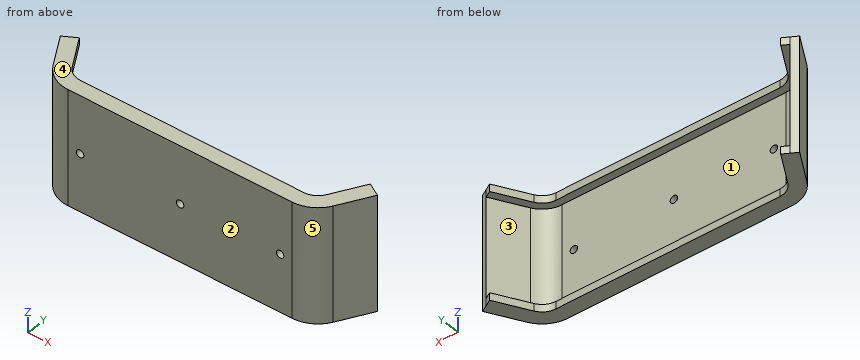
Autodesk Inventor part; units mm, degrees
ref_plane "Work Plane2" through (0, 0, 20) normal (0, 0, 1) x (1, 0, 0)
ref_plane "YZ Plane" through (0, 0, 0) normal (1, 0, 0) x (0, 1, 0)
ref_plane "XZ Plane" through (0, 0, 0) normal (0, 1, 0) x (-1, 0, 0)
sketch "Sketch1" plane through (0, 0, 0) normal (0, 0, 1) x (1, 0, 0)
  arc A0 (-53.4049, 8) -> (-44.7446, 3) centre (-44.7446, 13) ccw
  line L0 (-44.7446, 3) -> (44.7446, 3)
  arc A1 (44.7446, 3) -> (53.4049, 8) centre (44.7446, 13) ccw
  line L1 (53.4049, 8) -> (60.8108, 20.8273)
  line L2 (-60.8108, 20.8273) -> (-53.4049, 8)
  line L3 (63.4088, 19.3273) -> (56.003, 6.5)
  arc A2 (44.7446, 0) -> (56.003, 6.5) centre (44.7446, 13) ccw
  line L4 (44.7446, 0) -> (-44.7446, 0)
  arc A3 (-56.003, 6.5) -> (-44.7446, 0) centre (-44.7446, 13) ccw
  line L5 (-56.003, 6.5) -> (-63.4088, 19.3273)
  line L6 (-63.4088, 19.3273) -> (-60.8108, 20.8273)
  line L7 (-60.8108, 20.8273) -> (60.8108, 20.8273) construction
  line L8 (-63.4088, 19.3273) -> (63.4088, 19.3273) construction
  line L9 (60.8108, 20.8273) -> (63.4088, 19.3273)
  point P0 (0, 0)
  point P1 (0, 0)
extrude "Extrusion1" add sketch "Sketch1" along normal blind 40
sketch "Sketch2" plane through (-44.7446, 0, 0) normal (0, -1, 0) x (1, 0, 0)
  line L0 (89.4893, 0) -> (0, 0)
  line L1 (-11.2583, 0) -> (-11.2583, 40)
  line L2 (0, 0) -> (0, 40)
  line L3 (89.4893, 0) -> (89.4893, 40)
  point P0 (44.7446, 0)
  point P1 (4.7446, 20)
  point P2 (44.7446, 20)
  point P3 (84.7446, 20)
  point P4 (44.7446, 0)
  point P5 (-11.2583, 20)
  dimension "d3" = 40
  dimension "d4" = 40
  dimension "d30" = 4.7447
  dimension "d31" = 4.7447
hole "Hole1" at (-40, 0, 20) at (0, 0, 20) at (40, 0, 20) direction (0, 1, 0) diameter 3 end through all
sketch "Sketch3" plane through (-44.7446, 0, 0) normal (0, -1, 0) x (1, 0, 0)
  circle A0 centre (44.7446, 20) radius 1.5
  line L0 (89.4893, 0) -> (0, 0)
  line L1 (0, 0) -> (0, 40)
  line L2 (0, 20) -> (89.4893, 20) construction
  line L3 (89.4893, 0) -> (89.4893, 40)
  point P0 (44.7446, 0)
  point P1 (24.7446, 7)
  point P2 (64.7446, 7)
  point P3 (24.7446, 33)
  point P4 (64.7446, 33)
  dimension "d12" = 20
  dimension "d13" = 20
  dimension "d14" = 7
hole "Hole2" [suppressed]
ref_plane "Work Plane2" through (0, 0, 20) normal (0, 0, 1) x (1, 0, 0)
sketch "Sketch5" plane through (0, 0, 40) normal (0, 0, 1) x (1, 0, 0)
  arc A0 (-53.4049, 8) -> (-44.7446, 3) centre (-44.7446, 13) ccw
  line L0 (-53.4049, 8) -> (-60.8108, 20.8273)
  line L1 (-60.8108, 20.8273) -> (-63.4088, 19.3273)
  line L2 (-63.4088, 19.3273) -> (-56.003, 6.5)
  arc A1 (-56.003, 6.5) -> (-44.7446, 0) centre (-44.7446, 13) ccw
  line L3 (-44.7446, 0) -> (44.7446, 0)
  arc A2 (44.7446, 0) -> (56.003, 6.5) centre (44.7446, 13) ccw
  line L4 (56.003, 6.5) -> (63.4088, 19.3273)
  line L5 (63.4088, 19.3273) -> (60.8108, 20.8273)
  line L6 (60.8108, 20.8273) -> (53.4049, 8)
  arc A3 (44.7446, 3) -> (53.4049, 8) centre (44.7446, 13) ccw
  line L7 (44.7446, 3) -> (-44.7446, 3)
  point P0 (0, 0)
extrude "Extrusion3" add sketch "Sketch5" along normal blind 0.25
sketch "Sketch6" plane through (0, 0, 40.25) normal (0, 0, 1) x (1, 0, 0)
  arc A0 (-53.4049, 8) -> (-44.7446, 3) centre (-44.7446, 13) ccw
  line L0 (-53.4049, 8) -> (-60.8108, 20.8273)
  line L1 (-60.8108, 20.8273) -> (-63.4088, 19.3273)
  line L2 (-63.4088, 19.3273) -> (-56.003, 6.5)
  arc A1 (-56.003, 6.5) -> (-44.7446, 0) centre (-44.7446, 13) ccw
  line L3 (-44.7446, 0) -> (44.7446, 0)
  arc A2 (44.7446, 0) -> (56.003, 6.5) centre (44.7446, 13) ccw
  line L4 (56.003, 6.5) -> (63.4088, 19.3273)
  line L5 (63.4088, 19.3273) -> (60.8108, 20.8273)
  line L6 (60.8108, 20.8273) -> (53.4049, 8)
  arc A3 (44.7446, 3) -> (53.4049, 8) centre (44.7446, 13) ccw
  line L7 (44.7446, 3) -> (-44.7446, 3)
  arc A4 (-50.8068, 9.5) -> (-44.7446, 6) centre (-44.7446, 13) ccw
  line L8 (-50.8068, 9.5) -> (-58.2127, 22.3273)
  line L9 (58.2127, 22.3273) -> (50.8068, 9.5)
  arc A5 (44.7446, 6) -> (50.8068, 9.5) centre (44.7446, 13) ccw
  line L10 (44.7446, 6) -> (-44.7446, 6)
  line L11 (-63.4088, 19.3273) -> (-60.8108, 20.8273)
  line L12 (-63.4088, 19.3273) -> (-58.2127, 22.3273)
  line L13 (63.4088, 19.3273) -> (58.2127, 22.3273)
  dimension "d27" = 3
extrude "Extrusion4" add sketch "Sketch6" along normal blind 3
mirror "Mirror2" about plane through (0, 0, 20) normal (0, 0, 1) of "Extrusion3", "Extrusion4"
properties part number "Drill Helper v 1"
The model under review builds one solid part; all positions refer to its coordinate system, in mm. Face numbers are marked on the shaded views. A direction names the side the tool comes from. Round coordinates to 2 decimals unless told otherwise and drop trailing zeros. Order: outer loops, then holes, each group sorted by start corner. A loop starts at its lowest first (then second) coordinate and runs counter-clockwise, first axis right, second up. Notation, with made-up numbers: (-20.5, -6) -> (15.5, -6) arc R12 cw to (15.5, 11) -> close; hole circle Ø7 at (-3, 71.5). An arc over 180 degrees is marked (long way). Use CSV: the item, a comma, the result in double quotes. Start each with the question number.
(1) Consider section A-A on z = 20. Write out the cut boundary in (x, y), and give its area (3 significant figures).
(2) Consider section B-B on x = 0. Write out the cut boundary in (y, z).
(3) Insertion check: pin 1 (1.5 mm diameter, centred on x = -29.5, z = 22.5, fed in from +Y); pin 2 (3 mm diameter, centred on y = 9, z = 36, fed in from +X); pin 3 (4 mm diameter, centred on y = 17.5, z = 29.5, fed in from -X). Each pin has a flat end and moves straight along its axis. Give the tip position at first contact, or say it passes through.
(4) Consider section D-D on y = 13.5. Write out the cut boundary in (x, z).
(5) Tool access review of the marked faces 1 and 2: name each direction out of +Z, -Z, +X, -X, +Y, -Y from which nothing blocks a thin tool from reaching the whole face with its end or side.
(6) Consider section C-C on x = -15.5. Write out the cut boundary in (y, z), and give its area (4 significant figures).
(7) Wall thickness on probe 1 along Z at (x, y) = (-40, 1.6); probe 2 along Z at (x, y) = (48, 4); probe 3 along X at (y, z) = (1.2, 20): over which ranges is each line inside the solid? List them lowest first. Write a range as from..to.
(8) Mouldability with a two-part tool opening along X and no side actions: class the marked faces 3, 4 and 5 as pulls with the +X half, pulls with the -X half, needs draft (parallel to the pull), parting line crosses it, or undercut.
Responses:
1,outline,"(-63.41, 19.33) -> (-56, 6.5) arc R13 ccw to (-44.74, 0) -> (-41.5, 0) -> (-41.5, 3) -> (-44.74, 3) arc R10 cw to (-53.4, 8) -> (-60.81, 20.83) -> close; (-38.5, 0) -> (-1.5, 0) -> (-1.5, 3) -> (-38.5, 3) -> close; (1.5, 0) -> (38.5, 0) -> (38.5, 3) -> (1.5, 3) -> close; (41.5, 0) -> (44.74, 0) arc R13 ccw to (56, 6.5) -> (63.41, 19.33) -> (60.81, 20.83) -> (53.4, 8) arc R10 cw to (44.74, 3) -> (41.5, 3) -> close"
1,area,"403 mm²"
2,outline,"(0, -3.25) -> (6, -3.25) -> (6, -0.25) -> (3, -0.25) -> (3, 18.5) -> (0, 18.5) -> close; (0, 21.5) -> (3, 21.5) -> (3, 40.25) -> (6, 40.25) -> (6, 43.25) -> (0, 43.25) -> close"
3,pin 1,"y = 3"
3,pin 2,"x = 58.31"
3,pin 3,"x = -63.41"
4,outline,"(-60.04, -3.25) -> (-53.12, -3.25) -> (-53.12, -0.25) -> (-56.58, -0.25) -> (-56.58, 40.25) -> (-53.12, 40.25) -> (-53.12, 43.25) -> (-60.04, 43.25) -> close; (53.12, -3.25) -> (60.04, -3.25) -> (60.04, 43.25) -> (53.12, 43.25) -> (53.12, 40.25) -> (56.58, 40.25) -> (56.58, -0.25) -> (53.12, -0.25) -> close"
5,face 1,"+Y"
5,face 2,"+Z, -Z, +X, -X, -Y"
6,outline,"(0, -3.25) -> (6, -3.25) -> (6, -0.25) -> (3, -0.25) -> (3, 40.25) -> (6, 40.25) -> (6, 43.25) -> (0, 43.25) -> close"
6,area,"157.5 mm²"
7,probe 1,"-3.25..18.5, 21.5..43.25"
7,probe 2,"-3.25..-0.25, 40.25..43.25"
7,probe 3,"-50.2..-41.5, -38.5..-1.5, 1.5..38.5, 41.5..50.2"
8,face 3,"undercut"
8,face 4,"needs draft"
8,face 5,"pulls with the +X half"
